from build123d import *

# Parameters (mm, degrees)
SKETCH1_R           = 1.7
BOSS_EXTRUDE1_DEPTH = 12.7
SKETCH2_W           = 6.35
SKETCH2_H           = 10.16
CUT_EXTRUDE1_DEPTH  = 20.32
CHAMFER1_SIZE       = 0.5


with BuildPart() as part:
    # Sketch1 → Boss-Extrude1 (new body)
    with BuildSketch(Plane.XY):
        with BuildLine():
            Line((2.54, 47.625), (7.62, 47.625))
            ThreePointArc((7.62, 47.625), (9.416051224, 46.881051224), (10.16, 45.085))
            Line((10.16, 45.085), (10.16, 40.005))
            ThreePointArc((10.16, 40.005), (9.416051224, 38.208948776), (7.62, 37.465))
            Line((7.62, 37.465), (5.08, 37.465))
            ThreePointArc((5.08, 37.465), (3.283948776, 36.721051224), (2.54, 34.925))
            Line((2.54, 34.925), (2.54, -43.815))
            ThreePointArc((2.54, -43.815), (1.424076836, -46.509076836), (-1.27, -47.625))
            Line((-1.27, -47.625), (-2.54, -47.625))
            Line((-2.54, -47.625), (-2.54, -45.085))
            Line((-2.54, -45.085), (-5.08, -45.085))
            Line((-5.08, -45.085), (-5.08, -37.465))
            Line((-5.08, -37.465), (-2.54, -37.465))
            Line((-2.54, -37.465), (-2.54, -20.955))
            ThreePointArc((-2.54, -20.955), (-2.911974388, -20.056974388), (-3.81, -19.685))
            Line((-3.81, -19.685), (-6.985, -19.685))
            ThreePointArc((-6.985, -19.685), (-10.795, -15.875), (-6.985, -12.065))
            Line((-6.985, -12.065), (-3.81, -12.065))
            ThreePointArc((-3.81, -12.065), (-2.911974388, -11.693025612), (-2.54, -10.795))
            Line((-2.54, -10.795), (-2.54, 43.815))
            ThreePointArc((-2.54, 43.815), (-1.424076836, 46.509076836), (1.27, 47.625))
            Line((1.27, 47.625), (2.54, 47.625))
        make_face()
        with Locations((-6.985, -15.875)):
            Circle(SKETCH1_R, mode=Mode.SUBTRACT)
    extrude(amount=BOSS_EXTRUDE1_DEPTH)

    # Sketch2 → Cut-Extrude1 (cut)
    with BuildSketch(Plane.ZY.offset(2.54)):
        with Locations((9.525, -15.875)):
            Rectangle(SKETCH2_W, SKETCH2_H)
    extrude(amount=CUT_EXTRUDE1_DEPTH, mode=Mode.SUBTRACT)

    # Chamfer1
    chamfer1_edges = [part.edges().sort_by_distance(p)[0] for p in [
        (-3.81, -45.085, 0),
        (-5.08, -41.275, 0),
        (-3.81, -37.465, 0),
        (-2.54, -29.21, 0),
        (-2.911974388, -20.056974388, 0),
        (-5.3975, -19.685, 0),
        (-10.795, -15.875, 0),
        (-5.3975, -12.065, 0),
        (-2.911974388, -11.693025612, 0),
        (-2.54, 16.51, 0),
        (-1.424076836, 46.509076836, 0),
        (4.445, 47.625, 0),
        (9.416051224, 46.881051224, 0),
        (10.16, 42.545, 0),
        (9.416051224, 38.208948776, 0),
        (6.35, 37.465, 0),
        (3.283948776, 36.721051224, 0),
        (2.54, -4.445, 0),
        (1.424076836, -46.509076836, 0),
        (-1.905, -47.625, 0),
        (-2.54, -46.355, 0),
        (-8.685, -15.875, 0),
    ]]
    chamfer(chamfer1_edges, length=CHAMFER1_SIZE)


solid = part.part
Input: part model. Units: mm. Frame: model coordinates. A direction names the side the tool comes from. Give positions to 0.01 mm unless a question says otherwise; leave off trailing zeros. Loops run counter-clockwise (first coordinate to the right, second up) from the corner with the lowest first, then second, coordinate; pieces in that order, holes last. Notation, with made-up numbers: M 26.5,43 L 64.5,43 A21 ccw 64.5,73 Z; hole C -18.5,-39 d2. An arc over 180 degrees is marked long. Use CSV: the item, a comma, the result in double quotes.
(1) Section B-B, the plane y = -25.5. Return loops of the section in (x, z).
Outcome:
outline,"M -2.54,0.5 L -2.04,0 L 2.04,0 L 2.54,0.5 L 2.54,12.7 L -2.54,12.7 Z"
(2) Set-up query: faces 1 (the face through (6, 37.465, 7)), 2 (the face through (-4, -37.465, 7)), 3 (the face through (-2.54, -46, 7)). Return all of +Z, -Z, +X, -X, +Y, -Y with unobstructed straight access to the full face (end or side cutting, diameter ignored); none if empty.
Outcome:
face 1,"+Z, -Z, +X, -Y"
face 2,"+Z, -Z, -X"
face 3,"+Z, -Z, -X, -Y"
(3) Pull-direction query (Y, two-part tool) for faces 4 (the face through (1.454, -46.479, 6.515)), 5 (the face through (-2.78, -11.84, 0.3)), 6 (the face through (1, 1, 12.7)), 7 (the face through (-2.76, -19.93, 0.3)); classes: pulls with the +Y half, pulls with the -Y half, needs draft (parallel to the pull), parting line crosses it, or undercut.
Outcome:
face 4,"pulls with the -Y half"
face 5,"pulls with the +Y half"
face 6,"needs draft"
face 7,"undercut"
(4) Material intervals for L1, parallel to Y at x = -5.25, z = 0.75 (3 decimals); L2, parallel to X at y = 40.5, z = 1.75; L3, parallel to X at y = 10.5, z = 1, sorted ascending. Write a range as [from, to].
Outcome:
L1,"y = [-19.685, -12.065]"
L2,"x = [-2.54, 10.16]"
L3,"x = [-2.54, 2.54]"
(5) Section A-A, the plane z = 7.75. Return loops of the section in (x, y) (3 decimals).
Outcome:
outline,"M -5.08,-45.085 L -2.54,-45.085 L -2.54,-47.625 L -1.27,-47.625 A3.81 ccw 2.54,-43.815 L 2.54,34.925 A2.54 cw 5.08,37.465 L 7.62,37.465 A2.54 ccw 10.16,40.005 L 10.16,45.085 A2.54 ccw 7.62,47.625 L 1.27,47.625 A3.81 ccw -2.54,43.815 L -2.54,-37.465 L -5.08,-37.465 Z"
(6) Section C-C, the plane x = 6.75. Return loops of the section in (y, z) (3 decimals), plus the area to 3 significant figures.
Outcome:
outline,"M 37.465,0.5 L 37.965,0 L 47.125,0 L 47.625,0.5 L 47.625,12.7 L 37.465,12.7 Z"
area,"129 mm²"
(7) Section D-D, the plane z = 2.5. Return loops of the section in (x, y) (3 decimals).
Outcome:
outline,"M -6.985,-19.685 L -3.81,-19.685 A1.27 cw -2.54,-20.955 L -2.54,-37.465 L -5.08,-37.465 L -5.08,-45.085 L -2.54,-45.085 L -2.54,-47.625 L -1.27,-47.625 A3.81 ccw 2.54,-43.815 L 2.54,34.925 A2.54 cw 5.08,37.465 L 7.62,37.465 A2.54 ccw 10.16,40.005 L 10.16,45.085 A2.54 ccw 7.62,47.625 L 1.27,47.625 A3.81 ccw -2.54,43.815 L -2.54,-10.795 A1.27 cw -3.81,-12.065 L -6.985,-12.065 A3.81 ccw Z; hole C -6.985,-15.875 d3.4"
(8) Pin query (flat end, axial travel): P1, Ø9, axis at x = -7, y = -15, coming from the +Z side; P2, Ø3, axis at x = -6.5, z = 7, coming from the -Y side (3 decimals); P3, Ø1, axis at x = -4.5, z = 3, coming from the +Y side (3 decimals); P4, Ø2, axis at y = -46, z = 8, coming from the -X side. Return the tip coordinate at first contact, or that it passes through.
Outcome:
P1,"stops at z = 12.7"
P2,"stops at y = -45.085"
P3,"stops at y = -12.065"
P4,"stops at x = -5.08"
